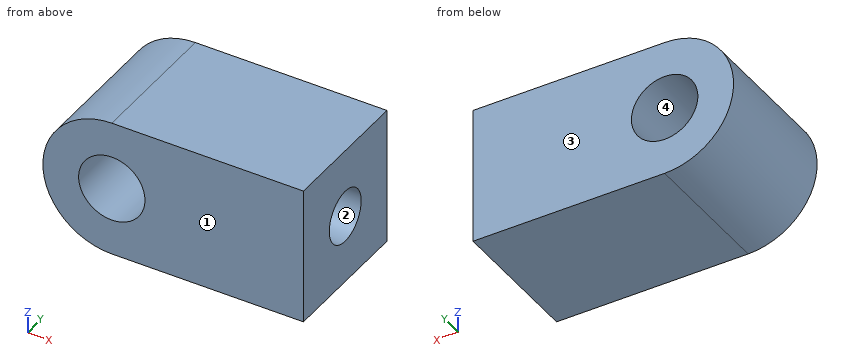
```python
from build123d import *

# Parameters (mm, degrees)
F0_R     = 6.5
F1_DEPTH = 13.5
F3_D     = 10.3
F3_DEPTH = 25.25
F3_TIP   = 3.094432188


with BuildPart() as f1:
    # F0 (on Front) → F1 (new body, symmetric)
    with BuildSketch(Plane.XZ):
        with BuildLine():
            ThreePointArc((-37.525, -13.5), (-27.979058454, -9.545941546), (-24.025, 0))
            ThreePointArc((-24.025, 0), (-27.979058454, 9.545941546), (-37.525, 13.5))
            ThreePointArc((-37.525, 13.5), (-51.025, 0), (-37.525, -13.5))
        make_face()
        with Locations((-37.525, 0)):
            Circle(F0_R, mode=Mode.SUBTRACT)
        with BuildLine():
            ThreePointArc((-37.525, 13.5), (-27.979058454, 9.545941546), (-24.025, 0))
            ThreePointArc((-24.025, 0), (-27.979058454, -9.545941546), (-37.525, -13.5))
            Line((-37.525, -13.5), (0, -13.5))
            Line((0, -13.5), (0, 13.5))
            Line((0, 13.5), (-37.525, 13.5))
        make_face()
    extrude(amount=F1_DEPTH, both=True)

    # F3
    with Locations(Plane.YZ):
        with Locations((0, 0)):
            Hole(F3_D / 2, depth=F3_DEPTH)
            with Locations((0, 0, -(F3_DEPTH + F3_TIP / 2))):  # 118° drill point
                Cone(0, F3_D / 2, F3_TIP, mode=Mode.SUBTRACT)


solid = f1.part
```
Here's how the part is built. I have some questions about the finished solid (model axes, mm). Face numbers are marked on the shaded views. Give positions to 0.01 mm unless a question says otherwise; leave off trailing zeros. Loops run counter-clockwise (first coordinate to the right, second up) from the corner with the lowest first, then second, coordinate; pieces in that order, holes last. Notation, with made-up numbers: (-33, -24.75) -> (-22, -24.75) arc R12 cw to (-22, -5.75) -> close; hole circle Ø5 at (-5, 6). An arc over 180 degrees is marked (long way). Use one line per item in the form item = value. Start each with the question number.
1) Thinking about a two-plate mould opening in Y: for the marked faces 1, 2, 3 and 4, which applies, +Y half, -Y half, draft (parallel to the pull), parting line (faces both ways), or undercut?
2) For P1, Ø4, axis at y = 9, z = -6.5, coming from the -X side; P2, Ø8, axis at x = -37.525, z = 0, coming from the +Y side; P3, Ø5, axis at y = 2, z = 0.5, coming from the +X side; P4, Ø5, axis at y = -10, z = 6, coming from the -X side, each with a flat end and sliding along its axis, tell me the tip position at first contact or that it passes through.
3) Imagine slicing it at A-A (x = -40). Please give me the cut outline in (y, z).
4) Imagine slicing it at D-D (z = -9). Please give me the cut outline in (x, y), then the cut area to 3 significant figures.
5) Imagine slicing it at B-B (y = -7). Please give me the cut outline in (x, z) (3 decimals), then the cut area to 3 significant figures.
6) Please list where these lines run through material, in increasing order: line 1 along Y through (x, z) = (-13, 0); line 2 along X through (y, z) = (-7.75, 3.5).
7) Imagine slicing it at C-C (x = -12). Please give me the cut outline in (y, z).
Check values:
q1.face_1 = -Y half
q1.face_2 = undercut
q1.face_3 = +Y half
q1.face_4 = draft
q2.P1 = -50.25
q2.P2 = through
q2.P3 = -25.6
q2.P4 = -50.56
q3.outline = (-13.5, -13.27) -> (13.5, -13.27) -> (13.5, -6.01) -> (-13.5, -6.01) -> close; (-13.5, 6.01) -> (13.5, 6.01) -> (13.5, 13.27) -> (-13.5, 13.27) -> close
q4.outline = (-47.59, -13.5) -> (0, -13.5) -> (0, 13.5) -> (-47.59, 13.5) -> close
q4.area = 1,280 mm^2
q5.outline = (-37.525, -13.5) -> (0, -13.5) -> (0, 13.5) -> (-37.525, 13.5) arc R13.5 ccw to start; hole circle Ø13 at (-37.525, 0)
q5.area = 1,170 mm^2
q6.line_1 = -13.5 to -5.15, 5.15 to 13.5
q6.line_2 = -50.56 to -43, -32.05 to 0
q7.outline = (-13.5, -13.5) -> (13.5, -13.5) -> (13.5, 13.5) -> (-13.5, 13.5) -> close; hole circle Ø10.3 at (0, 0)
